For this review, take the finished solid that the model builds, in its own axes (mm). A direction names the side the tool comes from. Round coordinates to 2 decimals unless told otherwise and drop trailing zeros. Write each loop counter-clockwise with the first axis right and the second up, starting at its lowest first coordinate (ties: lowest second). Pieces come first, ordered by that corner, then holes. Notation, with made-up numbers: (-36.5, 58.25) -> (-22.5, 58.25) arc R13 cw to (-22.5, 78.25) -> close; hole circle Ø2 at (83, 68). An arc over 180 degrees is marked (long way). Answer in a Markdown table with one row per item.
from build123d import *

# Parameters (mm, degrees)
SKETCH1_W                        = 68.600000001
SKETCH1_H                        = 113.65
BRACKETBASE_DEPTH                = 5
ARDUINOMOUNTINGHOLES_DEPTH       = 22
ARDUINOMOUNTINGHOLES_DEPTH_BACK  = 120.777809299
ARDUINOMOUNTINGHOLESSKETCH_R     = 1.25
F_9VBATTERYMOUNTINGHOLESSKETCH_R = 1.25
F_9VBATTERYMOUNTINGHOLES_DEPTH   = 20
LEGBRACKETMOUNTINGHOLESSKETCH_R  = 2
LEGBRACKETMOUNTINGHOLES_DEPTH    = 13
BACKSIDEMOUNTINGHOLESSKETCH_R    = 1.25
BACKSIDEMOUNTINGHOLES_DEPTH      = 24
COVER_START                      = -5
SKETCH2_R                        = 1.25
SKETCH2_R_2                      = 2
COVER_DEPTH                      = 5
SKETCH3_W                        = 64
SKETCH3_H                        = 92
SKETCH3_W_2                      = 58
SKETCH3_H_2                      = 86
BREADBOARDCAVITY_DEPTH           = 10
SKETCH4_W                        = 64
SKETCH4_H                        = 10
CUT_EXTRUDE1_DEPTH               = 125.514820906
SKETCH5_R                        = 2.875
TOGGLESWITCHHOLE_DEPTH           = 10
SKETCH6_R                        = 2.125
CUT_EXTRUDE2_DEPTH               = 10


with BuildPart() as part:
    # Sketch1 → bracketBase (new body)
    with BuildSketch(Plane.XY):
        with Locations((34.3, 41.235000001)):
            Rectangle(SKETCH1_W, SKETCH1_H)
    extrude(amount=BRACKETBASE_DEPTH)

    # arduinoMountingHolesSketch → arduinoMountingHoles (cut, two sides: drawn at the far end of the back side and taken through both)
    with BuildSketch(Plane.XY.offset(-ARDUINOMOUNTINGHOLES_DEPTH_BACK)):
        with Locations((2.54, 2.280000001)):
            Circle(ARDUINOMOUNTINGHOLESSKETCH_R)
        with Locations((2.54, 30.450000001)):
            Circle(ARDUINOMOUNTINGHOLESSKETCH_R)
        with Locations((54.600000001, 35.270000001)):
            Circle(ARDUINOMOUNTINGHOLESSKETCH_R)
        with Locations((53.350000001, -13.049999999)):
            Circle(ARDUINOMOUNTINGHOLESSKETCH_R)
    extrude(amount=ARDUINOMOUNTINGHOLES_DEPTH + ARDUINOMOUNTINGHOLES_DEPTH_BACK, mode=Mode.SUBTRACT)

    # 9VbatteryMountingHolesSketch → 9VbatteryMountingHoles (cut)
    with BuildSketch(Plane.XY):
        with Locations((8.625000001, 86.060000001)):
            Circle(F_9VBATTERYMOUNTINGHOLESSKETCH_R)
        with Locations(Location((59.975000001, 86.060000001, 0), (0, 0, 180))):
            Circle(F_9VBATTERYMOUNTINGHOLESSKETCH_R)
        with Locations(Location((8.625000001, 42.810000001, 0), (0, 0, 180))):
            Circle(F_9VBATTERYMOUNTINGHOLESSKETCH_R)
        with Locations((59.975000001, 42.810000001)):
            Circle(F_9VBATTERYMOUNTINGHOLESSKETCH_R)
    extrude(amount=F_9VBATTERYMOUNTINGHOLES_DEPTH, mode=Mode.SUBTRACT)

    # legBracketMountingHolesSketch → legBracketMountingHoles (cut)
    with BuildSketch(Plane.XY):
        with Locations((29.202551646, 94.560000001)):
            Circle(LEGBRACKETMOUNTINGHOLESSKETCH_R)
        with Locations(Location((39.397448356, 94.560000001, 0), (0, 0, 180))):
            Circle(LEGBRACKETMOUNTINGHOLESSKETCH_R)
    extrude(amount=LEGBRACKETMOUNTINGHOLES_DEPTH, mode=Mode.SUBTRACT)

    # backsideMountingHolesSketch → backsideMountingHoles (cut)
    with BuildSketch(Plane.XY):
        with Locations((2.875000001, 94.560000001)):
            Circle(BACKSIDEMOUNTINGHOLESSKETCH_R)
        with Locations(Location((65.725000001, 94.560000001, 0), (0, 0, 180))):
            Circle(BACKSIDEMOUNTINGHOLESSKETCH_R)
        with Locations((65.725000001, -12.089999999)):
            Circle(BACKSIDEMOUNTINGHOLESSKETCH_R)
        with Locations(Location((2.875000001, -12.089999999, 0), (0, 0, 180))):
            Circle(BACKSIDEMOUNTINGHOLESSKETCH_R)
    extrude(amount=BACKSIDEMOUNTINGHOLES_DEPTH, mode=Mode.SUBTRACT)

    # Sketch2 → cover (add)
    with BuildSketch(Plane.XY.offset(5).offset(COVER_START)):
        with Locations((53.350000001, -13.049999999)):
            Circle(SKETCH2_R)
        with Locations((2.54, 2.280000001)):
            Circle(SKETCH2_R)
        with Locations((2.54, 30.450000001)):
            Circle(SKETCH2_R)
        with Locations((54.600000001, 35.270000001)):
            Circle(SKETCH2_R)
        with Locations((59.975000001, 42.810000001)):
            Circle(SKETCH2_R)
        with Locations((8.625000001, 42.810000001)):
            Circle(SKETCH2_R)
        with Locations((59.975000001, 86.060000001)):
            Circle(SKETCH2_R)
        with Locations((39.397448356, 94.560000001)):
            Circle(SKETCH2_R_2)
        with Locations((29.202551646, 94.560000001)):
            Circle(SKETCH2_R_2)
        with Locations((8.625000001, 86.060000001)):
            Circle(SKETCH2_R)
    extrude(amount=COVER_DEPTH)

    # Sketch3 → breadBoardCavity (add)
    with BuildSketch(Plane.XY.offset(5)):
        with Locations((34.300000001, 41.235000001)):
            Rectangle(SKETCH3_W, SKETCH3_H)
        with Locations((34.300000001, 41.235000001)):
            Rectangle(SKETCH3_W_2, SKETCH3_H_2, mode=Mode.SUBTRACT)
    breadboardcavity = extrude(amount=BREADBOARDCAVITY_DEPTH)

    # Mirror1: breadBoardCavity across plane
    add(breadboardcavity.mirror(Plane.XY.offset(2.5)))

    # Sketch4 → Cut-Extrude1 (cut, through all)
    with BuildSketch(Plane(origin=(0, 87.235000001, 0), x_dir=(1, 0, 0), z_dir=(0, 1, 0))):
        with Locations((34.300000001, -10)):
            Rectangle(SKETCH4_W, SKETCH4_H)
    extrude(amount=-CUT_EXTRUDE1_DEPTH, mode=Mode.SUBTRACT)

    # Sketch5 → toggleSwitchHole (cut)
    with BuildSketch(Plane(origin=(0, 0, 0), x_dir=(-1, 0, 0), z_dir=(0, 0, -1))):
        with Locations((-34.300000001, 91.810031891)):
            Circle(SKETCH5_R)
    extrude(amount=-TOGGLESWITCHHOLE_DEPTH, mode=Mode.SUBTRACT)

    # Sketch6 → Cut-Extrude2 (cut)
    with BuildSketch(Plane(origin=(0, 0, 0), x_dir=(-1, 0, 0), z_dir=(0, 0, -1))):
        with Locations((-39.397448351, -12.089999999)):
            Circle(SKETCH6_R)
        with Locations(Location((-29.202551651, -12.089999999, 0), (0, 0, 180))):
            Circle(SKETCH6_R)
    extrude(amount=-CUT_EXTRUDE2_DEPTH, mode=Mode.SUBTRACT)


solid = part.part
1) Mouldability with a two-part tool opening along X and no side actions: class faces 5 (the flat face through (68.6, 40, 2)), 6 (the flat face through (63.3, 41, -5)), 7 (the flat face through (34, -15.59, 2)) as pulls with the +X half, pulls with the -X half, needs draft (parallel to the pull), parting line crosses it, or undercut.
Solved:
| item | result |
|---|---|
| face 5 | pulls with the +X half |
| face 6 | undercut |
| face 7 | needs draft |
2) Consider section C-C on y = -12.09. State the section outline as (x, z) points (3 decimals), then the cut area to 4 significant figures.
Solved:
| item | result |
|---|---|
| outline | (0, 0) -> (1.625, 0) -> (1.625, 5) -> (0, 5) -> close; (4.125, 0) -> (27.078, 0) -> (27.078, 5) -> (4.125, 5) -> close; (31.328, 0) -> (37.272, 0) -> (37.272, 5) -> (31.328, 5) -> close; (41.522, 0) -> (64.475, 0) -> (64.475, 5) -> (41.522, 5) -> close; (66.975, 0) -> (68.6, 0) -> (68.6, 5) -> (66.975, 5) -> close |
| area | 275.5 mm² |
3) For faces 1 (the flat face through (34, 42, 0)), 2 (the flat face through (66.3, 41, -5)), 3 (the flat face through (34, -4.765, -5)), 4 (the cylindrical face through (66.88, -12.57, 2.46)), list the 3-axis set-ups (+Z, -Z, +X, -X, +Y, -Y) from which the entire face can be reached by the end or side of a thin tool; tool diameter is ignored.
Solved:
| item | result |
|---|---|
| face 1 | -Z |
| face 2 | -Z, +X, +Y, -Y |
| face 3 | -Z, +X, -X, -Y |
| face 4 | +Z, -Z |
4) For line 1 (Y direction, x = 63, z = -3.75) (3 decimals); line 2 (X direction, y = 69, z = -1.5); line 3 (Y direction, x = 29.5, z = 3.5), list the stretches that pass through material, from the lowest coordinate up. Write a range as [from, to].
Solved:
| item | result |
|---|---|
| line 1 | [-4.765, -1.765], [84.235, 87.235] |
| line 2 | [2.3, 5.3], [63.3, 66.3] |
| line 3 | [-15.59, -14.19], [-9.99, 98.06] |
5) Consider section A-A on z = -8.25. State the section outline as (x, y) points (3 decimals).
Solved:
| item | result |
|---|---|
| outline | (2.3, -4.765) -> (66.3, -4.765) -> (66.3, 87.235) -> (2.3, 87.235) -> close; hole (5.3, -1.765) -> (63.3, -1.765) -> (63.3, 84.235) -> (5.3, 84.235) -> close |
6) Consider section D-D on y = 45. State the section outline as (x, z) points.
Solved:
| item | result |
|---|---|
| outline | (0, 0) -> (2.3, 0) -> (2.3, -10) -> (5.3, -10) -> (5.3, 0) -> (63.3, 0) -> (63.3, -10) -> (66.3, -10) -> (66.3, 0) -> (68.6, 0) -> (68.6, 5) -> (0, 5) -> close |
7) Consider section B-B on x = 34.3. State the section outline as (y, z) points (3 decimals).
Solved:
| item | result |
|---|---|
| outline | (-15.59, 0) -> (-4.765, 0) -> (-4.765, -10) -> (-1.765, -10) -> (-1.765, 0) -> (84.235, 0) -> (84.235, -10) -> (87.235, -10) -> (87.235, 0) -> (88.935, 0) -> (88.935, 5) -> (-15.59, 5) -> close; (94.685, 0) -> (98.06, 0) -> (98.06, 5) -> (94.685, 5) -> close |
8) Clearance check with flat-ended pins moving along their axes: pin 1 Ø5 at (x, z) = (28, -7.5) entering from -Y (3 decimals); pin 2 Ø5 at (x, z) = (25, -4.5) entering from +Y (3 decimals); pin 3 Ø4 at (x, y) = (39.4, -12.09) entering from +Z; pin 4 Ø3 at (y, z) = (51.5, -4) entering from +X. State where each tip first meets the part, or that it passes through.
Solved:
| item | result |
|---|---|
| pin 1 | y = -4.765 |
| pin 2 | y = 87.235 |
| pin 3 | through |
| pin 4 | x = 66.3 |
